Here's how the part is built. I have some questions about the finished solid (model axes, mm). A direction names the side the tool comes from. Coordinates: 2 decimals unless noted, no trailing zeros. Order: outer loops, then holes, each group sorted by start corner. A loop starts at its lowest first (then second) coordinate and runs counter-clockwise, first axis right, second up. Notation, with made-up numbers: (8.5, 39.25) -> (64.5, 39.25) arc R14 ccw to (64.5, 66.25) -> close; hole circle Ø1 at (81.5, 30). An arc over 180 degrees is marked (long way). One line per item, written item: value. Start each with the question number.
Autodesk Inventor part; units mm, degrees
ref_plane "Work Plane1" through (12.1861, 4.5831, 113.4) normal (0, 0, -1) x (0, 1, 0)
ref_plane "YZ Plane" through (0, 0, 0) normal (1, 0, 0) x (0, 1, 0)
ref_plane "XZ Plane" through (0, 0, 0) normal (0, 1, 0) x (-1, 0, 0)
sketch "Sketch1" plane through (0, 0, 0) normal (0, 0, 1) x (1, 0, 0)
  arc A0 (12.2, 9) -> (9.2, 12) centre (9.2, 9) ccw
  line L0 (12.7, 12) -> (9.2, 12)
  line L1 (12.7, 12) -> (17.8, 6)
  line L2 (17.8, 6) -> (17.8, -32.6)
  line L3 (17.8, -32.6) -> (12.7, -38.6)
  line L4 (12.7, -38.6) -> (-12.7, -38.6)
  line L5 (-12.7, -38.6) -> (-17.8, -32.6)
  line L6 (-17.8, -32.6) -> (-17.8, 6)
  line L7 (-17.8, 6) -> (-12.7, 12)
  line L8 (-9.2, 12) -> (-12.7, 12)
  arc A1 (-9.2, 12) -> (-12.2, 9) centre (-9.2, 9) ccw
  line L9 (-12.2, -30) -> (-12.2, 9)
  arc A2 (-12.2, -30) -> (-9.2, -33) centre (-9.2, -30) ccw
  line L10 (9.2, -33) -> (-9.2, -33)
  arc A3 (9.2, -33) -> (12.2, -30) centre (9.2, -30) ccw
  line L11 (12.2, 9) -> (12.2, -30)
  circle A4 centre (-15, -29.5) radius 1.35
  circle A5 centre (15, -29.5) radius 1.35
  circle A6 centre (-8.5, -35.8) radius 1.35
  circle A7 centre (-15, -12.5) radius 1.35
  circle A8 centre (-15, 4.5) radius 1.35
  circle A9 centre (8.5, -35.8) radius 1.35
  circle A10 centre (15, -12.5) radius 1.35
  circle A11 centre (15, 4.5) radius 1.35
  line L12 (12.2, -16) -> (12.2, 29.9608)
  line L13 (29.7534, 60.3642) -> (34.7534, 60.3642)
  line L14 (34.7534, 60.3642) -> (34.7534, 53.3642)
  line L15 (34.7534, 53.3642) -> (17.8, 24)
  line L16 (17.8, 24) -> (17.8, -16)
  line L17 (12.2, -16) -> (17.8, -16)
  circle A12 centre (15, -12.5) radius 1.35
  circle A13 centre (15, 4.5) radius 1.35
  line L18 (12.2, 29.9608) -> (29.7534, 60.3642)
  point P0 (0, 0)
  dimension "d1" = 2.7
  dimension "d2" = 2.7
  dimension "d3" = 5.6
  dimension "d4" = 3.5
  dimension "d5" = 40
  dimension "d6" = 30
  dimension "d7" = 7
  dimension "d9" = 5
extrude "Extrusion1" add sketch "Sketch1" along normal blind 5 contours L12 L0 L1 L2 L17 L11 | L12 L18 L13 L14 L15 L16 L1 L0
sketch "Sketch2" plane through (0, 0, 5) normal (0, 0, 1) x (1, 0, 0)
  line L0 (34.7534, 60.3642) -> (34.7534, 53.3642)
  line L1 (29.7534, 60.3642) -> (34.7534, 60.3642)
  line L2 (34.7534, 60.3642) -> (29.7534, 60.3642)
  line L3 (34.7534, 60.3642) -> (29.7534, 60.3642)
  line L4 (29.7534, 60.3642) -> (25.712, 53.3642)
  line L5 (29.7534, 60.3642) -> (12.2, 29.9608)
  line L6 (34.7534, 53.3642) -> (25.712, 53.3642)
  line L7 (34.7534, 53.3642) -> (34.7534, 60.3642)
  point P0 (0, 0)
ref_plane "Work Plane1" through (12.1861, 4.5831, 113.4) normal (0, 0, -1) x (0, 1, 0)
extrude "Extrusion2" add sketch "Sketch2" along normal up to surface (108.4 mm away)
sketch "Sketch3" plane through (25.712, 53.3642, 113.4) normal (0, 0, 1) x (1, 0, 0)
  line L0 (9.0415, 7) -> (4.0415, 7)
  line L1 (4.0415, 7) -> (0, 0)
  line L2 (0, 0) -> (9.0415, 0)
  line L3 (9.0415, 0) -> (9.0415, 7)
  circle A0 centre (-10.712, -48.8642) radius 1.35
  circle A1 centre (-10.712, -65.8642) radius 1.35
  line L4 (-13.512, -23.4034) -> (-13.512, -69.3642)
  line L5 (4.0415, 7) -> (-13.512, -23.4034)
  line L6 (9.0415, 7) -> (4.0415, 7)
  line L7 (9.0415, 0) -> (9.0415, 7)
  line L8 (-7.912, -29.3642) -> (9.0415, 0)
  line L9 (-7.912, -69.3642) -> (-7.912, -29.3642)
  line L10 (-13.512, -69.3642) -> (-7.912, -69.3642)
  point P0 (-25.712, -53.3642)
extrude "Extrusion3" add sketch "Sketch3" against normal blind 5 contours L8 L9 L10 L4 L5 L2
properties part number "Alça" material "Aluminum-6061"
Q1. Imagine slicing it at B-B (x = 15). Write out the boundary of the cut face in (y, z), plus the area to 3 significant figures.
Q2. For P1, Ø2.5, axis at x = 29.5, z = 73, coming from the -Y side; P2, Ø4, axis at y = 4.5, z = 2.5, coming from the +X side, each with a flat end and sliding along its axis, tell me the tip position at first contact or that it passes through.
Q3. For faces 1 (the face through (15, -16, 111)), 2 (the face through (17.6, 24, 5)), 3 (the face through (17.8, 4, 2)), which set-ups out of +Z, -Z, +X, -X, +Y, -Y let a thin tool reach every point of the face, with its end or its side?
Q4. I need wall thicknesses on line 1 (Y direction, x = 15, z = 112.1); line 2 (Y direction, x = 34, z = 16.5); line 3 (Z direction, x = 14.5, y = 25). Which ranges of each line are inside material? Lowest first, please.
Q5. Imagine slicing it at A-A (y = 7.5). Write out the boundary of the cut face in (x, z), plus the area to 3 significant figures.
Q6. Imagine slicing it at D-D (z = 82.5). Write out the boundary of the cut face in (x, y).
Q7. Imagine slicing it at C-C (x = 21). Write out the boundary of the cut face in (y, z), plus the area to 3 significant figures.
Q8. If we mould it in two halves opening along Y, with no side actions, what happens to faces 4 (the face through (13.65, 4.56, 110.94)), 5 (the face through (26.16, 38.48, 110.94)), 6 (the face through (12.2, 7, 2))? For each: +Y half, -Y half, draft (parallel to the pull), parting line (faces both ways), or undercut.
Completed:
1. outline: (-16, 0) -> (-13.85, 0) -> (-13.85, 5) -> (-16, 5) -> close; (-16, 108.4) -> (-13.85, 108.4) -> (-13.85, 113.4) -> (-16, 113.4) -> close; (-11.15, 0) -> (3.15, 0) -> (3.15, 5) -> (-11.15, 5) -> close; (-11.15, 108.4) -> (3.15, 108.4) -> (3.15, 113.4) -> (-11.15, 113.4) -> close; (5.85, 0) -> (34.81, 0) -> (34.81, 5) -> (5.85, 5) -> close; (5.85, 108.4) -> (34.81, 108.4) -> (34.81, 113.4) -> (5.85, 113.4) -> close
1. area: 454 mm2
2. P1: stops at y = 53.36
2. P2: stops at x = 17.8
3. face 1: +Z, -Z, +X, -X, -Y
3. face 2: +X, -X, -Y
3. face 3: +Z, -Z, +X, -Y
4. line 1: y = -16 to -13.85, -11.15 to 3.15, 5.85 to 34.81
4. line 2: y = 53.36 to 60.36
4. line 3: z = 0 to 5, 108.4 to 113.4
5. outline: (12.2, 0) -> (17.8, 0) -> (17.8, 5) -> (12.2, 5) -> close; (12.2, 108.4) -> (17.8, 108.4) -> (17.8, 113.4) -> (12.2, 113.4) -> close
5. area: 56.0 mm2
6. outline: (25.71, 53.36) -> (34.75, 53.36) -> (34.75, 60.36) -> (29.75, 60.36) -> close
7. outline: (29.54, 0) -> (45.2, 0) -> (45.2, 5) -> (29.54, 5) -> close; (29.54, 108.4) -> (45.2, 108.4) -> (45.2, 113.4) -> (29.54, 113.4) -> close
7. area: 157 mm2
8. face 4: undercut
8. face 5: -Y half
8. face 6: draft
